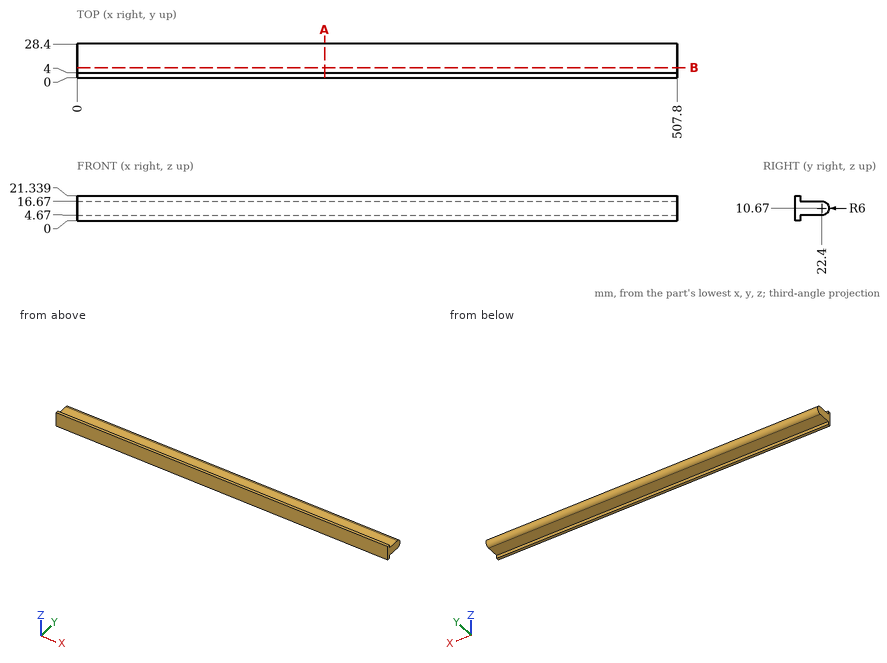
Print and shaded views of the part. All mm, measured from the part's lowest x, y and z. Round coordinates to 2 decimals unless told otherwise and drop trailing zeros. Loops run counter-clockwise (first coordinate to the right, second up) from the corner with the lowest first, then second, coordinate; pieces in that order, holes last. Notation, with made-up numbers: M -38.5,20 L 6.5,20 A4 cw 6.5,26 Z; hole C 42.5,-32 d9. An arc over 180 degrees is marked long. One line per question, with ' | ' between items.
1) Flat gauge pins, fed straight in: pin 1 (14.5 mm diameter, centred on x = 257.5, y = 14, fed in from +Z); pin 2 (3.5 mm diameter, centred on x = 278, z = 1.5, fed in from +Y); pin 3 (6 mm diameter, centred on x = 414, y = 15, fed in from -Z); pin 4 (1.5 mm diameter, centred on y = 8.5, z = 3.5, fed in from -X). Where does each tip first touch, or does it go through?
Solved:
pin 1: stops at z = 16.67 | pin 2: stops at y = 4 | pin 3: stops at z = 4.67 | pin 4: passes through
2) Band-saw the part on A-A (x = 209.5). Give the cut face in (y, z), then the cut area to 3 significant figures.
Solved:
outline: M 0,0 L 4,0 L 4,4.67 L 22.4,4.67 A6 ccw 22.4,16.67 L 4,16.67 L 4,21.34 L 0,21.34 Z | area: 363 mm²
3) Drill centre lines: line 1 along Z through (x, y) = (309, 21); line 2 along Y through (x, z) = (263, 19.5); line 3 along Y through (x, z) = (278, 12.75). Where is each one in solid material? Low to high.
Solved:
line 1: z = 4.67 to 16.67 | line 2: y = 0 to 4 | line 3: y = 0 to 28.03
4) Band-saw the part on B-B (y = 8.5). Give the cut face in (x, z), then the cut area to 3 significant figures.
Solved:
outline: M 0,4.67 L 507.8,4.67 L 507.8,16.67 L 0,16.67 Z | area: 6,090 mm²
